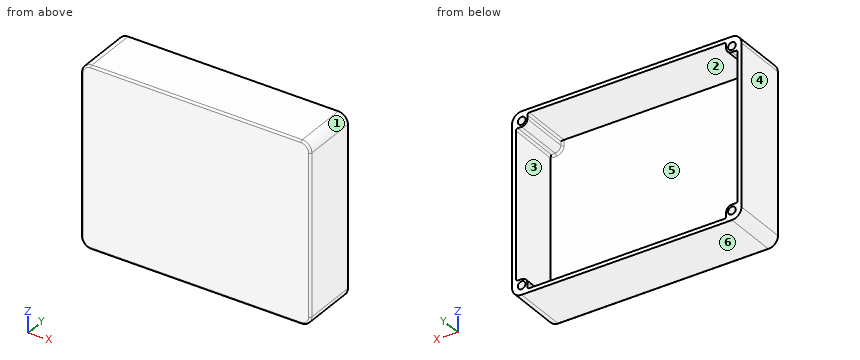
Autodesk Inventor part; units mm, degrees
ref_plane "YZ Plane" through (0, 0, 0) normal (1, 0, 0) x (0, 1, 0)
ref_plane "XZ Plane" through (0, 0, 0) normal (0, 1, 0) x (-1, 0, 0)
ref_plane "XY Plane" through (0, 0, 0) normal (0, 0, 1) x (1, 0, 0)
sketch "Esquisse1" plane through (0, 0, 0) normal (0, 1, 0) x (-1, 0, 0)
  line L0 (60, 47) -> (-60, 47)
  line L1 (-60, 47) -> (-60, -47)
  line L2 (-60, -47) -> (60, -47)
  line L3 (60, -47) -> (60, 47)
  line L4 (60, 47) -> (-60, -47) construction
  line L5 (-60, 47) -> (60, -47) construction
  line L6 (60, -47) -> (52, -47)
  line L7 (52, -47) -> (52, -39)
  line L8 (52, -39) -> (60, -39)
  line L9 (60, -39) -> (60, -47)
  line L10 (-60, -47) -> (-52, -47)
  line L11 (-52, -47) -> (-52, -39)
  line L12 (-52, -39) -> (-60, -39)
  line L13 (-60, -39) -> (-60, -47)
  line L14 (60, 47) -> (52, 47)
  line L15 (52, 47) -> (52, 39)
  line L16 (52, 39) -> (60, 39)
  line L17 (60, 39) -> (60, 47)
  line L18 (-60, 47) -> (-52, 47)
  line L19 (-52, 47) -> (-52, 39)
  line L20 (-52, 39) -> (-60, 39)
  line L21 (-60, 39) -> (-60, 47)
  circle A0 centre (-55, -42.115) radius 2
  line L22 (0, -47.6968) -> (0, 50.167) construction
  line L23 (81.8074, 0) -> (-86.221, 0) construction
  circle A1 centre (55, -42.115) radius 2
  circle A2 centre (-55, 42.115) radius 2
  circle A3 centre (55, 42.115) radius 2
  line L24 (58, -47) -> (58, 47)
  line L25 (60, 45) -> (-60, 45)
  line L26 (-60, -45) -> (60, -45)
  line L27 (-58, -47) -> (-58, 47)
  point P0 (0, 0)
  point P1 (-58, 39)
  point P2 (-58, -39)
  point P3 (-52, -45)
  point P4 (52, -45)
  point P5 (58, -39)
  point P6 (58, 39)
  point P7 (52, 45)
  point P8 (-52, 45)
  dimension "d0" = 120
  dimension "d1" = 94
  dimension "d2" = 8
  dimension "d3" = 8
  dimension "d4" = 8
  dimension "d5" = 8
  dimension "d6" = 8
  dimension "d8" = 4
  dimension "d9" = 55
  dimension "d10" = 42.115
  dimension "d11" = 8
  dimension "d12" = 2
  dimension "d13" = 2
  dimension "d14" = 2
  dimension "d15" = 2
extrude "Extrusion1" add sketch "Esquisse1" along normal blind 2 contours L15 L16 L24 L8 L7 L26 L11 L12 L27 L20 L19 L25
extrude "Extrusion2" add sketch "Esquisse1" along normal blind 29.1 contours L3 L25 L24 L0 | L24 L25 L15 L0 | L3 L16 L24 L25 | L15 L25 L19 L0 | L24 L16 L15 L25 | L3 L8 L24 L16 | L19 L25 L27 L0 | L3 L26 L24 L8 | L27 L25 L1 L0 | L19 L20 L27 L25 | L24 L26 L7 L8 | L3 L2 L24 L26 | L27 L20 L1 L25 | L24 L2 L7 L26 | L27 L12 L1 L20 | L7 L2 L11 L26 | L27 L26 L1 L12 | L12 L11 L26 L27 | L11 L2 L27 L26 | L27 L2 L1 L26
fillet "Congé1" radius 5 4 edges at (-60, 14.55, 47) (-60, 14.55, -47) (60, 14.55, -47) (60, 14.55, 47)
fillet "Congé2" radius 3 4 edges at (-52, 15.55, -39) (-52, 15.55, 39) (52, 15.55, -39) (52, 15.55, 39)
fillet "Congé3" radius 1 16 edges at (-58, 15.55, -39) (-52, 15.55, -45) (-52, 2, -43.5) (-56.5, 2, -39) (56.5, 2, -39) (52, 2, -43.5) (52, 15.55, -45) (58, 15.55, -39) (58, 15.55, 39) (52, 15.55, 45) (52, 2, 43.5) (56.5, 2, 39) (-56.5, 2, 39) (-52, 2, 43.5) (-58, 15.55, 39) (-52, 15.55, 45)
extrude "Extrusion3" add sketch "Esquisse1" along normal blind 19.1 contours A0 | A1 | A2 | A3
thread "Filetage1"
thread "Filetage2"
thread "Filetage3"
thread "Filetage4"
fillet "Congé4" radius 1 4 edges at (0, 0, 47) (60, 0, 0) (0, 0, -47) (-60, 0, 0)
sketch "Esquisse2" plane through (0, 29.1, 0) normal (0, 1, 0) x (1, 0, 0)
  arc A0 (55, -47) -> (60, -42) centre (55, -42) ccw
  line L0 (60, -42) -> (60, 42)
  arc A1 (60, 42) -> (55, 47) centre (55, 42) ccw
  line L1 (55, 47) -> (-55, 47)
  arc A2 (-55, 47) -> (-60, 42) centre (-55, 42) ccw
  line L2 (-60, 42) -> (-60, -42)
  arc A3 (-60, -42) -> (-55, -47) centre (-55, -42) ccw
  line L3 (-55, -47) -> (55, -47)
  circle A4 centre (55, 42.115) radius 2
  circle A5 centre (55, -42.115) radius 2
  circle A6 centre (-55, 42.115) radius 2
  circle A7 centre (-55, -42.115) radius 2
  arc A8 (55, -39) -> (52, -42) centre (55, -42) ccw
  line L4 (52, -42) -> (52, -44)
  arc A9 (51, -45) -> (52, -44) centre (51, -44) ccw
  line L5 (51, -45) -> (-51, -45)
  arc A10 (-52, -44) -> (-51, -45) centre (-51, -44) ccw
  line L6 (-52, -44) -> (-52, -42)
  arc A11 (-52, -42) -> (-55, -39) centre (-55, -42) ccw
  line L7 (-55, -39) -> (-57, -39)
  arc A12 (-58, -38) -> (-57, -39) centre (-57, -38) ccw
  line L8 (-58, -38) -> (-58, 38)
  arc A13 (-57, 39) -> (-58, 38) centre (-57, 38) ccw
  line L9 (-57, 39) -> (-55, 39)
  arc A14 (-55, 39) -> (-52, 42) centre (-55, 42) ccw
  line L10 (-52, 42) -> (-52, 44)
  arc A15 (-51, 45) -> (-52, 44) centre (-51, 44) ccw
  line L11 (-51, 45) -> (51, 45)
  arc A16 (52, 44) -> (51, 45) centre (51, 44) ccw
  line L12 (52, 44) -> (52, 42)
  arc A17 (52, 42) -> (55, 39) centre (55, 42) ccw
  line L13 (55, 39) -> (57, 39)
  arc A18 (58, 38) -> (57, 39) centre (57, 38) ccw
  line L14 (58, 38) -> (58, -38)
  arc A19 (57, -39) -> (58, -38) centre (57, -38) ccw
  line L15 (57, -39) -> (55, -39)
  point P0 (0, 0)
properties part number "Boitier_aluminium"
Input: part model. Units: mm. Frame: model coordinates. Face numbers are marked on the shaded views. A direction names the side the tool comes from. Round coordinates to 2 decimals unless told otherwise and drop trailing zeros. Order: outer loops, then holes, each group sorted by start corner. A loop starts at its lowest first (then second) coordinate and runs counter-clockwise, first axis right, second up. Notation, with made-up numbers: (73, -15) - (122, -15) arc R32 cw to (122, 14) - close; hole circle Ø8 at (-39, 78). An arc over 180 degrees is marked (long way). Use a Markdown table: item, result.
1. Section D-D on y = 24.25. State how many separate pieces and enclosed holes the cut face has, then the cut area to 3 significant figures.
Evaluation:
| item | result |
|---|---|
| separate pieces | 1 |
| enclosed holes | 5 |
| area | 906 mm^2 |
2. Material intervals for probe 1 along Z at (x, y) = (55, 22.25) (3 decimals); probe 2 along Z at (x, y) = (-49, 21.5); probe 3 along X at (y, z) = (16.75, -26), sorted ascending.
Evaluation:
| item | result |
|---|---|
| probe 1 | -47 to -44.115, -40.115 to -39, 39 to 40.115, 44.115 to 47 |
| probe 2 | -47 to -45, 45 to 47 |
| probe 3 | -60 to -58, 58 to 60 |
3. Access query for the marked faces 1 and 2. Directions: +Z, -Z, +X, -X, +Y, -Y. A direction counts if a zero-diameter tool reaches every point of the face in a straight line with its end or side. Return the directions, or none.
Evaluation:
| item | result |
|---|---|
| face 1 | +Z, +X, +Y, -Y |
| face 2 | +Y |
4. First-contact query: pin 1 (1.6 mm diameter, centred on y = 18.5, z = 43.5, fed in from +X); pin 2 (1.6 mm diameter, centred on y = 18, z = -43, fed in from -X); pin 3 (2 mm diameter, centred on x = -55.5, z = -42.5, fed in from +Y). Flat tips, straight axial feed; report the tip coordinate or a pass-through.
Evaluation:
| item | result |
|---|---|
| pin 1 | x = 59.95 |
| pin 2 | x = -60 |
| pin 3 | y = 19.1 |
5. Section B-B on x = -14. Return the cut outline in (y, z), then the cut area to 3 significant figures.
Evaluation:
| item | result |
|---|---|
| outline | (0, -46) arc R1 ccw to (1, -47) - (29.1, -47) - (29.1, -45) - (2, -45) - (2, 45) - (29.1, 45) - (29.1, 47) - (1, 47) arc R1 ccw to (0, 46) - close |
| area | 296 mm^2 |
6. Mould query, pull axis Z, two halves, no side actions, for the marked faces 3, 4, 5 and 6. Classes: +Z half, -Z half, draft (parallel to the pull), parting line (faces both ways), or undercut.
Evaluation:
| item | result |
|---|---|
| face 3 | undercut |
| face 4 | draft |
| face 5 | undercut |
| face 6 | -Z half |
7. Section C-C on z = 1.5. Return the cut outline in (x, y).
Evaluation:
| item | result |
|---|---|
| outline | (-60, 1) arc R1 ccw to (-59, 0) - (59, 0) arc R1 ccw to (60, 1) - (60, 29.1) - (58, 29.1) - (58, 2) - (-58, 2) - (-58, 29.1) - (-60, 29.1) - close |
